```python
from build123d import *

# Parameters (mm, degrees)
F1_DEPTH = 25.4


with BuildPart() as f1:
    # F0 (on Front) → F1 (new body, symmetric)
    with BuildSketch(Plane.XZ):
        with BuildLine():
            Line((35.127934, -4.863865), (26.841344, 36.20879))
            ThreePointArc((26.841344, 36.20879), (21.548443, 43.702101), (12.429882, 42.693947))
            Line((12.429882, 42.693947), (17.113609, -4.863865))
            ThreePointArc((17.113609, -4.863865), (26.120772, -13.431921), (35.127934, -4.863865))
        make_face()
        with BuildLine():
            ThreePointArc((34.767646, 29.363347), (33.665212, 36.098477), (26.841344, 36.20879))
            Line((26.841344, 36.20879), (35.127934, -4.863865))
            ThreePointArc((35.127934, -4.863865), (42.329691, -0.286863), (39.451364, 7.746161))
            ThreePointArc((39.451364, 7.746161), (44.526484, 11.832876), (45.936525, 18.194469))
            ThreePointArc((45.936525, 18.194469), (43.061412, 26.488234), (34.767646, 29.363347))
        make_face()
    extrude(amount=F1_DEPTH, both=True)


solid = f1.part
```
Check sheet for the modelled part. Datum: model origin and axes. Units: mm. Round coordinates to 2 decimals unless told otherwise and drop trailing zeros. Loops run counter-clockwise (first coordinate to the right, second up) from the corner with the lowest first, then second, coordinate; pieces in that order, holes last. Notation, with made-up numbers: (72, 47) -> (88, 47) arc R19 ccw to (88, 64) -> close; hole circle Ø10 at (-28.75, 38.5). An arc over 180 degrees is marked (long way). Write item = value, one per line. Start each with the question number.
1) Thickness scan on probe 1 along Z at (x, y) = (36, -16); probe 2 along X at (y, z) = (6.5, -11); probe 3 along X at (y, z) = (-23, 36). Record the ranges inside material, lowest first.
2) Sectioned sample at B-B, the plane z = -2. Record the cut outline in (x, y), plus the area to 3 significant figures.
3) Sectioned sample at C-C, the plane x = 31. Record the cut outline in (y, z), plus the area to 3 significant figures.
4) Sectioned sample at A-A, the plane y = -7.5. Record the cut outline in (x, z) (1 decimal).
5) Gauge pin test, flat ends, axial feed: pin 1 Ø8 at (x, y) = (32, -12.5) entering from -Z; pin 2 Ø5 at (y, z) = (-3.5, 33) entering from +X; pin 3 Ø1.5 at (x, y) = (22, 11) entering from -Z. Record the tip position at first contact, or that the pin passes through.
Results are:
q1.probe_1 = -4.9 to 29.43
q1.probe_2 = 19.96 to 32.28
q1.probe_3 = 13.09 to 33.78
q2.outline = (16.83, -25.4) -> (41.46, -25.4) -> (41.46, 25.4) -> (16.83, 25.4) -> close
q2.area = 1,250 mm^2
q3.outline = (-25.4, -12) -> (25.4, -12) -> (25.4, 37.33) -> (-25.4, 37.33) -> close
q3.area = 2,510 mm^2
q4.outline = (12.4, 42.7) -> (17.1, -4.9) arc R9 ccw to (35.1, -4.9) arc R6.8 ccw to (39.5, 7.7) arc R9.8 ccw to (45.9, 18.2) arc R10.1 ccw to (34.8, 29.4) arc R5.3 ccw to (26.8, 36.2) arc R9 ccw to start
q5.pin_1 = -13.23
q5.pin_2 = 35.51
q5.pin_3 = -12.78
